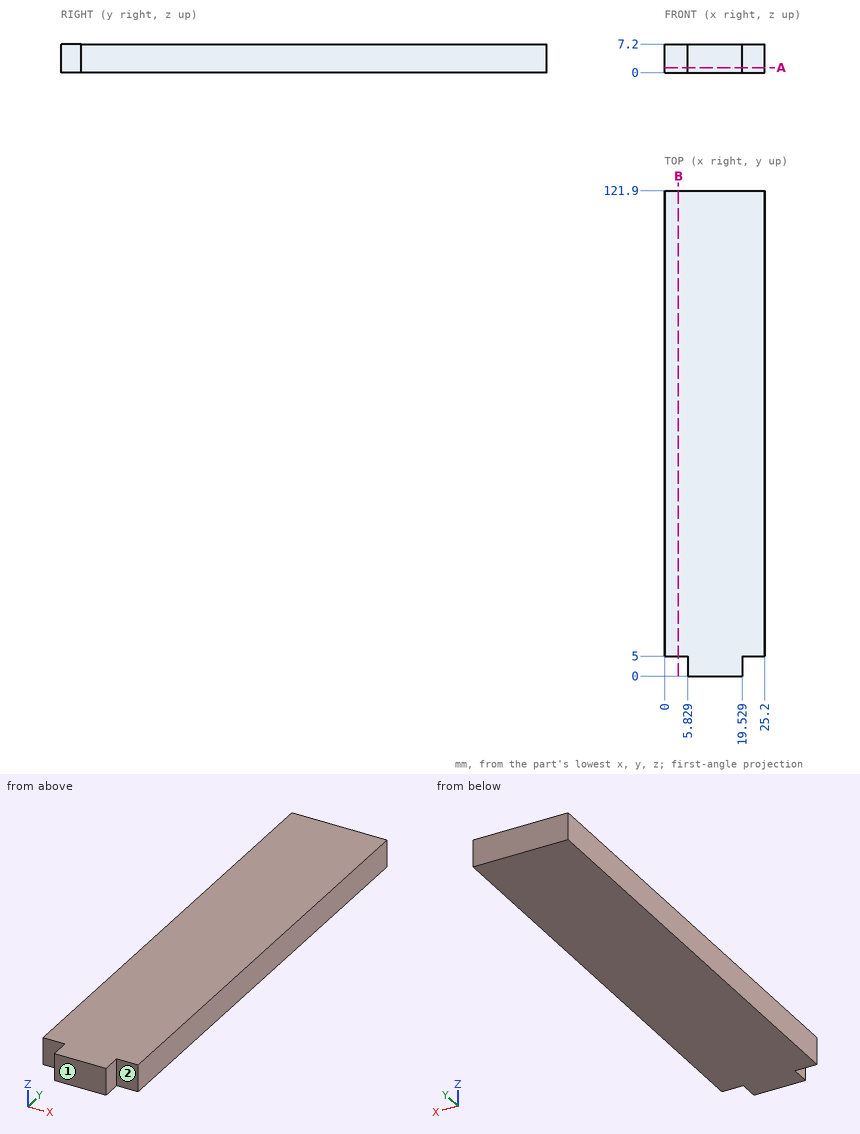
The drawing under review shows one solid part. Ordinate dimensions are in mm from its lowest x, y, z. A direction names the side the tool comes from. Round coordinates to 2 decimals unless told otherwise and drop trailing zeros. Write each loop counter-clockwise with the first axis right and the second up, starting at its lowest first coordinate (ties: lowest second). Pieces come first, ordered by that corner, then holes.
(1) Machinability: for the marked faces 1 and 2, which of the approach directions +Z, -Z, +X, -X, +Y, -Y give a long, thin tool a straight path to every point of the face, cutting with its end or side? Answer none if there is none.
(2) Insertion check: pin 1 (3 mm diameter, centred on x = 1.5, z = 2.5, fed in from -Y). The pin has a flat end and moves straight along its axis. Give the tip position at first contact, or say it passes through.
(3) Wall thickness on L1, parallel to Y at x = 21, z = 2.5: over which ranges is the line inside the solid? List them lowest first.
(4) We need section A-A on z = 1.25. Give the boundary of the cut face in (x, y).
(5) We need section B-B on x = 3.5. Give the boundary of the cut face in (y, z), and give its area (3 significant figures).
Findings below:
1. face 1: +Z, -Z, +X, -X, -Y
1. face 2: +Z, -Z, +X, -Y
2. pin 1: stops at y = 5
3. L1: y = 5 to 121.9
4. outline: (0, 5) - (5.83, 5) - (5.83, 0) - (19.53, 0) - (19.53, 5) - (25.2, 5) - (25.2, 121.9) - (0, 121.9) - close
5. outline: (5, 0) - (121.9, 0) - (121.9, 7.2) - (5, 7.2) - close
5. area: 842 mm2
